```python
from build123d import *

# Parameters (mm, degrees)
F1_DEPTH  = 1816.1
F2_R      = 4.953
F2_R_2    = 4.9657
F3_DEPTH  = 25.4
F4_R      = 4.953
F5_DEPTH  = 25.4
F6_R      = 4.953
F7_DEPTH  = 25.4
F8_W      = 23.9268
F8_H      = 96.8375
F8_W_2    = 24.13
F9_DEPTH  = 7.62
F10_R     = 4.953
F11_DEPTH = 25.4
F12_W     = 84.1502
F12_H     = 15.875
F12_W_2   = 88.9
F12_W_3   = 84.1248
F13_DEPTH = 25.273


with BuildPart() as f1:
    # F0 (on Front) → F1 (new body)
    with BuildSketch(Plane.XZ):
        Polygon((44.45, 0), (0, 0), (0, -57.15), (28.575, -57.15), (28.575, -41.275), (25.273, -41.275), (25.273, -53.848), (3.302, -53.848), (3.302, -3.302), (41.148, -3.302), (41.148, -19.05), (44.45, -19.05), align=None)
    extrude(amount=F1_DEPTH)

    # F2 (on face) → F3 (cut)
    with BuildSketch(Plane.XY):
        with Locations((23.622, -563.751269)):
            Circle(F2_R)
        with Locations((28.575, -1295.4)):
            Circle(F2_R_2)
    extrude(amount=-F3_DEPTH, mode=Mode.SUBTRACT)

    # F4 (on face) → F5 (cut)
    with BuildSketch(Plane(origin=(0, 0, 0), x_dir=(0, -1, 0), z_dir=(-1, 0, 0))):
        with Locations((14.2748, -38.8874)):
            Circle(F4_R)
        with Locations((65.0748, -38.8874)):
            Circle(F4_R)
        with Locations((531.7998, -38.8874)):
            Circle(F4_R)
        with Locations((582.5998, -38.8874)):
            Circle(F4_R)
        with Locations((1268.3998, -38.8874)):
            Circle(F4_R)
        with Locations((1319.1998, -38.8874)):
            Circle(F4_R)
        with Locations((1750.9998, -38.8874)):
            Circle(F4_R)
        with Locations((1801.7998, -38.8874)):
            Circle(F4_R)
    extrude(amount=-F5_DEPTH, mode=Mode.SUBTRACT)

    # F6 (on face) → F7 (cut)
    with BuildSketch(Plane(origin=(0, 0, 0), x_dir=(0, -1, 0), z_dir=(-1, 0, 0))):
        with Locations((833.4375, -28.575)):
            Circle(F6_R)
        with Locations((993.775, -28.575)):
            Circle(F6_R)
    extrude(amount=-F7_DEPTH, mode=Mode.SUBTRACT)

    # F8 (on face) → F9 (cut)
    with BuildSketch(Plane.XY):
        with Locations((11.9634, -150.01875)):
            Rectangle(F8_W, F8_H)
        with Locations((12.065, -1666.08125)):
            Rectangle(F8_W_2, F8_H)
        with Locations((12.065, -912.80615)):
            Rectangle(F8_W_2, F8_H)
    extrude(amount=-F9_DEPTH, mode=Mode.SUBTRACT)

    # F10 (on face) → F11 (cut)
    with BuildSketch(Plane(origin=(0, 0, 0), x_dir=(0, -1, 0), z_dir=(-1, 0, 0))):
        with Locations((150.0251, -31.9405)):
            Circle(F10_R)
        with Locations((912.8125, -26.9875)):
            Circle(F10_R)
        with Locations((1666.0876, -26.9875)):
            Circle(F10_R)
    extrude(amount=-F11_DEPTH, mode=Mode.SUBTRACT)

    # F12 (on face) → F13 (cut, through all)
    with BuildSketch(Plane.YZ.offset(28.575)):
        with Locations((-1774.0249, -49.2125)):
            Rectangle(F12_W, F12_H)
        with Locations((-1293.7998, -49.2125)):
            Rectangle(F12_W_2, F12_H)
        with Locations((-557.1998, -49.2125)):
            Rectangle(F12_W_2, F12_H)
        with Locations((-42.0624, -49.2125)):
            Rectangle(F12_W_3, F12_H)
    extrude(amount=-F13_DEPTH, mode=Mode.SUBTRACT)


solid = f1.part
```
Read the model definition and answer for the solid it produces. Units are mm, in the model's axes. A direction names the side the tool comes from. Coordinates: 2 decimals unless noted, no trailing zeros. Write each loop counter-clockwise with the first axis right and the second up, starting at its lowest first coordinate (ties: lowest second). Pieces come first, ordered by that corner, then holes. Notation, with made-up numbers: (60.25, -40) -> (108.25, -40) arc R26 cw to (108.25, -8) -> close; hole circle Ø5 at (86.25, 66.25). An arc over 180 degrees is marked (long way). Write item = value, one per line.
(1) Given pin 1 Ø8 at (x, z) = (10, -51.5) entering from -Y; pin 2 Ø14 at (y, z) = (-305, -46.5) entering from -X; pin 3 Ø2.5 at (x, y) = (43.5, -874.5) entering from -Z; pin 4 Ø4 at (y, z) = (-287, -37) entering from +X, each flat-ended and moving along its own axis, determine where each tip first touches the part or whether it passes through.
From the geometry:
pin_1 = -1731.95
pin_2 = 0
pin_3 = -19.05
pin_4 = 3.3
(2) For a pull along Z with two mould halves and no side action, classify faces 3 (the face through (16, 0, -3)), 4 (the face through (3.302, -895, -31)), 5 (the face through (14, -895, -57.15)) as +Z half, -Z half, draft (parallel to the pull), parting line (faces both ways), or undercut.
From the geometry:
face_3 = draft
face_4 = undercut
face_5 = -Z half
(3) Section B-B on y = -891 is taken. Write down the section's boundary in (x, z) (3 decimals).
From the geometry:
outline = (0, -57.15) -> (28.575, -57.15) -> (28.575, -41.275) -> (25.273, -41.275) -> (25.273, -53.848) -> (3.302, -53.848) -> (3.302, -7.62) -> (0, -7.62) -> close; (24.13, -3.302) -> (41.148, -3.302) -> (41.148, -19.05) -> (44.45, -19.05) -> (44.45, 0) -> (24.13, 0) -> close
(4) Straight lines are drawn through the part: L1, parallel to X at y = -1459, z = -51.5 (3 decimals); L2, parallel to Z at x = 26.5, y = -230 (3 decimals); L3, parallel to Z at x = 14.5, y = -1051. For each, find the intervals that lie inside material, in ascending order. Write a range as from..to.
From the geometry:
L1 = 0..3.302, 25.273..28.575
L2 = -57.15..-41.275, -3.302..0
L3 = -57.15..-53.85, -3.3..0
(5) Which of the six approach directions +Z, -Z, +X, -X, +Y, -Y give full straight-line access (tool end or side, diameter ignored) to faces 1 (the face through (0, -895, -28)), 2 (the face through (26, -895, -3.302))?
From the geometry:
face_1 = +Z, -Z, -X, +Y, -Y
face_2 = +Y, -Y
(6) Section A-A on x = 11 is taken. Write down the section's boundary in (y, z).
From the geometry:
outline = (-1816.1, -3.3) -> (-1714.5, -3.3) -> (-1714.5, 0) -> (-1816.1, 0) -> close; (-1731.95, -57.15) -> (-1338.25, -57.15) -> (-1338.25, -53.85) -> (-1731.95, -53.85) -> close; (-1617.66, -3.3) -> (-961.22, -3.3) -> (-961.22, 0) -> (-1617.66, 0) -> close; (-1249.35, -57.15) -> (-601.65, -57.15) -> (-601.65, -53.85) -> (-1249.35, -53.85) -> close; (-864.39, -3.3) -> (-198.44, -3.3) -> (-198.44, 0) -> (-864.39, 0) -> close; (-512.75, -57.15) -> (-84.12, -57.15) -> (-84.12, -53.85) -> (-512.75, -53.85) -> close; (-101.6, -3.3) -> (0, -3.3) -> (0, 0) -> (-101.6, 0) -> close
(7) Section C-C on y = -350.5 is taken. Write down the section's boundary in (x, z) (3 decimals).
From the geometry:
outline = (0, -57.15) -> (28.575, -57.15) -> (28.575, -41.275) -> (25.273, -41.275) -> (25.273, -53.848) -> (3.302, -53.848) -> (3.302, -3.302) -> (41.148, -3.302) -> (41.148, -19.05) -> (44.45, -19.05) -> (44.45, 0) -> (0, 0) -> close
